from build123d import *

# Parameters (mm, degrees)
F0_R     = 1.45
F1_DEPTH = 16
F2_R     = 2.9
F3_DEPTH = 2.4
F4_R     = 1
F5_W     = 1
F5_H     = 1
F6_DEPTH = 1.5


with BuildPart() as f1:
    # F0 (on Top) → F1 (new body)
    with BuildSketch(Plane.XY):
        Circle(F0_R)
    extrude(amount=F1_DEPTH)

    # F2 (on Top) → F3 (join)
    with BuildSketch(Plane.XY):
        Circle(F2_R)
    extrude(amount=-F3_DEPTH)

    # F4
    f4_edges = [f1.edges().sort_by_distance(p)[0] for p in [
        (-2.9, 0, -2.4),
    ]]
    fillet(f4_edges, radius=F4_R)

    # F5 (on face) → F6 (cut)
    with BuildSketch(Plane(origin=(0, 0, -2.4), x_dir=(1, 0, 0), z_dir=(0, 0, -1))):
        with Locations((1, 0)):
            Rectangle(F5_W, F5_H)
        Rectangle(F5_W, F5_H)
        with Locations((0, 1)):
            Rectangle(F5_W, F5_H)
        with Locations((-1, 0)):
            Rectangle(F5_W, F5_H)
        with Locations((0, -1)):
            Rectangle(F5_W, F5_H)
    extrude(amount=-F6_DEPTH, mode=Mode.SUBTRACT)


solid = f1.part
Part model, mm, in its own coordinate system. A direction names the side the tool comes from. Give positions to 0.01 mm unless a question says otherwise; leave off trailing zeros. Write each loop counter-clockwise with the first axis right and the second up, starting at its lowest first coordinate (ties: lowest second). Pieces come first, ordered by that corner, then holes.
1) Pin check, flat tips, straight feed: pin 1 (1.1 mm diameter, centred on y = 1, z = -1.5, fed in from -X); pin 2 (1.1 mm diameter, centred on x = -1, z = -2, fed in from -Y); pin 3 (1.1 mm diameter, centred on y = -1, z = -1.5, fed in from +X). Stop position of each tip, or through.
Resolved:
pin 1: stops at x = -2.86
pin 2: stops at y = -2.81
pin 3: stops at x = 2.86
2) Two-plate mould, pull along Y, no slides. Class faces 4 (the face through (-1.45, 0.06, 7.89)), 5 (the face through (1, -1, -2.4)), 6 (the face through (0, 1.5, -2)): released by +Y, released by -Y, zero draft, split by the parting line, or undercut.
Resolved:
face 4: split by the parting line
face 5: zero draft
face 6: undercut
3) Which spindle directions (+Z, -Z, +X, -X, +Y, -Y) get a long thin tool onto all of the face, cutting with end or side? Do faces 1 (the face through (-1.5, 0, -2)), 2 (the face through (0, 0, 16)), 3 (the face through (1.2, -1.2, 0)). Say none if no direction does.
Resolved:
face 1: -Z
face 2: +Z, +X, -X, +Y, -Y
face 3: +Z
4) Cut at C-C on z = 3. Write the cut outline in (x, y).
Resolved:
outline: circle Ø2.9 at (0, 0)
5) Probe L1, parallel to Z at x = -0.3, y = -1.6; L2, parallel to X at y = -0.75, z = -1.5; L3, parallel to Z at x = 1.05, y = 2.6. List the from-to ranges inside material, lowest first.
Resolved:
L1: z = -2.4 to 0
L2: x = -2.8 to -0.5, 0.5 to 2.8
L3: z = -1.83 to 0
6) Cut at A-A on y = 0. Write the cut outline in (x, z), then the cut area to 3 significant figures.
Resolved:
outline: (-2.9, -1.4) arc R1 ccw to (-1.9, -2.4) - (-1.5, -2.4) - (-1.5, -0.9) - (1.5, -0.9) - (1.5, -2.4) - (1.9, -2.4) arc R1 ccw to (2.9, -1.4) - (2.9, 0) - (1.45, 0) - (1.45, 16) - (-1.45, 16) - (-1.45, 0) - (-2.9, 0) - close
area: 55.4 mm2
